Part model, mm, in its own coordinate system. Face numbers are marked on the shaded views. Give positions to 0.01 mm unless a question says otherwise; leave off trailing zeros. Order: outer loops, then holes, each group sorted by start corner. A loop starts at its lowest first (then second) coordinate and runs counter-clockwise, first axis right, second up. Notation, with made-up numbers: (66.5, -5.5) -> (102.5, -5.5) arc R31 cw to (102.5, 33.5) -> close; hole circle Ø10 at (53.5, 22.5). An arc over 180 degrees is marked (long way). Write item = value, one per line. Start each with the question number.
Item 1: Pull direction Y, two halves, no side cores. Call the marked faces 1 and 2: +Y half, -Y half, draft (parallel to the pull), parting line (faces both ways), or undercut.
Item 2: Flat gauge pins, fed straight in: P1, Ø2, axis at x = -3, y = -16.5, coming from the +Z side; P2, Ø8.5, axis at x = -2.23, y = -14.88, coming from the +Z side; P3, Ø4, axis at y = -16, z = 5.5, coming from the -X side; P4, Ø2, axis at x = -2.23, y = -14.88, coming from the +Z side. Where does each tip first touch, or does it go through?
Item 3: Band-saw the part on A-A on z = 0. Write the cut outline in (x, y).
Item 4: Drill centre lines: line 1 along X through (y, z) = (-13, 16); line 2 along X through (y, z) = (-16, 6.5); line 3 along Z through (x, y) = (62, -7.5). Where is each one in solid material? Low to high.
Item 5: Band-saw the part on C-C on y = -2. Write the cut outline in (x, z).
Item 6: Band-saw the part on D-D on y = 17.5. Write the cut outline in (x, z).
Item 7: Band-saw the part on B-B on x = 57.5. Write the cut outline in (y, z).
Autodesk Inventor part; units mm, degrees
ref_plane "Plan de construction1" through (50, 0, -25) normal (0, 0, 1) x (1, 0, 0)
ref_plane "Plan de construction2" through (50, 0, 35) normal (0, 0, -1) x (-1, 0, 0)
ref_plane "YZ Plane" through (0, 0, 0) normal (1, 0, 0) x (0, 1, 0)
sketch "Esquisse1" plane through (0, 0, 0) normal (0, 1, 0) x (-1, 0, 0)
  line L0 (0, 0) -> (-100, 0)
  line L1 (-100, 0) -> (-100, -25)
  line L2 (-100, -25) -> (0, -25)
  line L3 (0, -25) -> (0, 0)
  arc A0 (0, -25) -> (25, 0) centre (0, 0) ccw
  line L4 (25, 0) -> (0, 0)
  line L5 (0, 0) -> (0, -25)
  line L6 (-100, 0) -> (-100, -25)
  arc A1 (-125, 0) -> (-100, -25) centre (-100, 0) ccw
  line L7 (-100, 0) -> (-125, 0)
  dimension "d1" = 25
  dimension "d2" = 100
revolve "Révolution1" add sketch "Esquisse1" angle 360 about axis through (0, 0, 0) along (1, 0, 0)
ref_plane "Plan de construction1" through (50, 0, -25) normal (0, 0, 1) x (1, 0, 0)
sketch "Esquisse2" plane through (50, 0, -25) normal (0, 0, 1) x (1, 0, 0)
  arc A0 (-50, 25) -> (-50, -25) centre (-50, 0) ccw
  line L0 (-50, 0) -> (-62.5, -21.6506)
  line L1 (-62.5, -21.6506) -> (-84.1506, -9.1506)
  line L2 (-84.1506, -9.1506) -> (-71.6506, 12.5)
  line L3 (-71.6506, 12.5) -> (-50, 0)
  line L4 (-50, 0) -> (-17.1432, 0)
  line L5 (-50, 0) -> (-6.6987, -25)
  line L6 (-6.6987, -25) -> (-19.1987, -46.6506)
  line L7 (-19.1987, -46.6506) -> (-62.5, -21.6506)
  line L8 (-62.5, -21.6506) -> (-50, 0)
  line L9 (-50, -25) -> (-50, 25) construction
  line L10 (-50, -25) -> (100.3384, -25) construction
  dimension "d8" = 120
extrude "Extrusion1" cut sketch "Esquisse2" along normal blind 30
ref_plane "Plan de construction2" through (50, 0, 35) normal (0, 0, -1) x (-1, 0, 0)
sketch "Esquisse3" plane through (50, 0, 35) normal (0, 0, -1) x (-1, 0, 0)
  line L0 (65.2228, -7.3769) -> (52.2324, -14.8769) construction
  circle A0 centre (52.2324, -14.8769) radius 1.7
  circle A1 centre (65.2228, -7.3769) radius 1.7
  line L1 (71.2132, 12.2474) -> (50, 0) construction
  line L2 (71.2132, 12.2474) -> (-7.2, -33.0245) construction
  line L3 (71.2132, 12.2474) -> (83.9867, -9.8769) construction
  dimension "d15" = 3.4
  dimension "d16" = 3.4
  dimension "d23" = 14
  dimension "d24" = 15
  dimension "d25" = 30
extrude "Extrusion2" cut sketch "Esquisse3" along normal blind 30
sketch "Esquisse4" plane through (50, 0, 35) normal (0, 0, -1) x (-1, 0, 0)
  circle A0 centre (65.2228, -7.3769) radius 1.7
  circle A1 centre (65.2228, -7.3769) radius 3.25
  circle A2 centre (52.2324, -14.8769) radius 1.7
  circle A3 centre (52.2324, -14.8769) radius 3.25
  point P0 (50, 0)
  dimension "d19" = 6.5
  dimension "d20" = 6.5
extrude "Extrusion3" cut sketch "Esquisse4" along normal blind 20
equation "\"d16\" = d15"
equation "\"d20\" = d19"
properties part number "P1704_002_mainDroite"
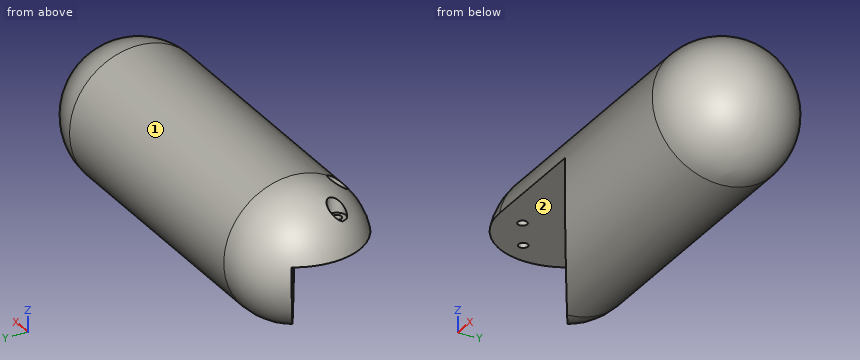
Values found:
q1.face_1 = parting line
q1.face_2 = draft
q2.P1 = 15
q2.P2 = 22.55
q2.P3 = -20.06
q2.P4 = through
q3.outline = (-21.65, 12.5) -> (0, 0) -> (43.3, -25) -> (100, -25) arc R25 ccw to (100, 25) -> (0, 25) arc R25 ccw to start
q4.line_1 = -14.14 to -4.89, 0.42 to 114.14
q4.line_2 = -18.08 to -3.51, -0.96 to 118.08
q4.line_3 = -23.85 to 23.85
q5.outline = (-24.41, 5) -> (3.46, 5) -> (3.46, -24.92) -> (100, -24.92) arc R24.92 ccw to (100, 24.92) -> (0, 24.92) arc R24.92 ccw to start
q6.outline = (0, -17.85) -> (100, -17.85) arc R17.85 ccw to (100, 17.85) -> (0, 17.85) arc R17.85 ccw to start
q7.outline = circle Ø50 at (0, 0)
